Answer from the drawing. Dimensions are ordinates in mm from the lowest x, y and z of the part. A direction names the side the tool comes from. Coordinates: 2 decimals unless noted, no trailing zeros. Loops run counter-clockwise (first coordinate to the right, second up) from the corner with the lowest first, then second, coordinate; pieces in that order, holes last.
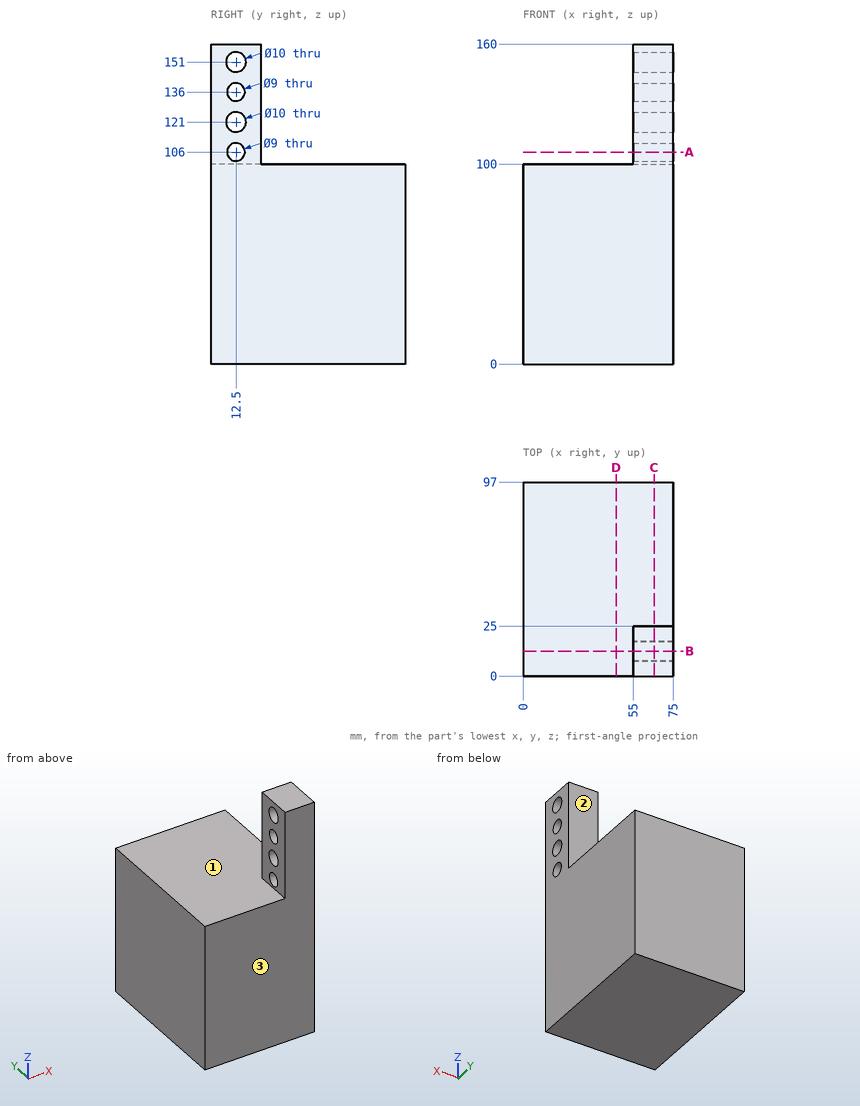
Item 1: A cutting plane is placed at C-C on x = 65.5. Determine the outline of the cut face in (y, z), then the cut area to 3 significant figures.
Numbers:
outline: (0, 0) - (97, 0) - (97, 100) - (25, 100) - (25, 160) - (0, 160) - close; hole circle Ø10 at (12.5, 121); hole circle Ø10 at (12.5, 151); hole circle Ø9 at (12.5, 106); hole circle Ø9 at (12.5, 136)
area: 10,900 mm2
Item 2: Given pin 1 (10 mm diameter, centred on x = 41, y = 77, fed in from +Z); pin 2 (6 mm diameter, centred on x = 61, z = 135, fed in from +Y); pin 3 (7.5 mm diameter, centred on y = 17.5, z = 119.5, fed in from -X), each flat-ended and moving along its own axis, determine where each tip first touches the part or whether it passes through.
Numbers:
pin 1: stops at z = 100
pin 2: stops at y = 25
pin 3: stops at x = 55
Item 3: A cutting plane is placed at D-D on x = 46.5. Determine the outline of the cut face in (y, z), then the cut area to 3 significant figures.
Numbers:
outline: (0, 0) - (97, 0) - (97, 100) - (0, 100) - close
area: 9,700 mm2
Item 4: Find the intervals of material crossed by line 1 along Z through (x, y) = (59.75, 12.5); line 2 along Y through (x, z) = (68, 136); line 3 along Z through (x, y) = (53, 21.5), in increasing order.
Numbers:
line 1: z = 0 to 101.5, 110.5 to 116, 126 to 131.5, 140.5 to 146, 156 to 160
line 2: y = 0 to 8, 17 to 25
line 3: z = 0 to 100
Item 5: A cutting plane is placed at B-B on y = 12.5. Determine the outline of the cut face in (x, z), then the cut area to 3 significant figures.
Numbers:
outline: (0, 0) - (75, 0) - (75, 101.5) - (55, 101.5) - (55, 100) - (0, 100) - close; (55, 110.5) - (75, 110.5) - (75, 116) - (55, 116) - close; (55, 126) - (75, 126) - (75, 131.5) - (55, 131.5) - close; (55, 140.5) - (75, 140.5) - (75, 146) - (55, 146) - close; (55, 156) - (75, 156) - (75, 160) - (55, 160) - close
area: 7,940 mm2
Item 6: Which of the six approach directions +Z, -Z, +X, -X, +Y, -Y give full straight-line access (tool end or side, diameter ignored) to the marked faces 1, 2 and 3?
Numbers:
face 1: +Z, -X, +Y
face 2: +Z, +X, -X, +Y
face 3: +Z, -Z, +X, -X, -Y
Item 7: A cutting plane is placed at A-A on z = 106. Determine the outline of the cut face in (x, y).
Numbers:
outline: (55, 0) - (75, 0) - (75, 8) - (55, 8) - close; (55, 17) - (75, 17) - (75, 25) - (55, 25) - close
